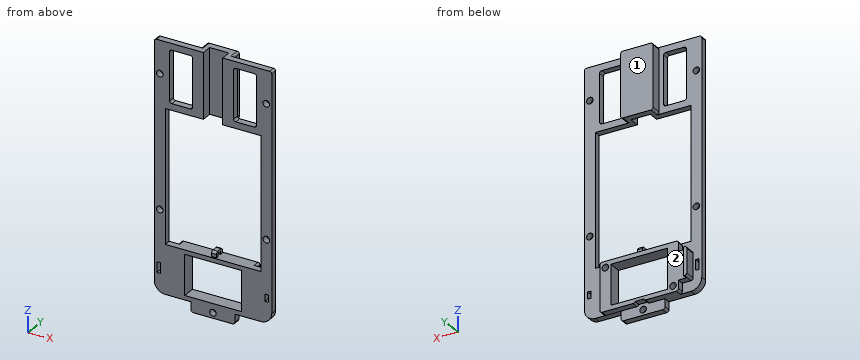
from build123d import *

# Parameters (mm, degrees)
BOSS_EXTRUDE1_DEPTH = 30
BOSS_EXTRUDE2_DEPTH = 3
SKETCH4_W           = 10.48
SKETCH4_H           = 24
CUT_EXTRUDE1_DEPTH  = 93.244717637
SKETCH5_R           = 1.5
CUT_EXTRUDE2_DEPTH  = 93.244717637
FILLET1_R           = 1
SKETCH7_W           = 26
SKETCH7_H           = 18.47
BOSS_EXTRUDE3_DEPTH = 3
SKETCH8_R           = 1.5
CUT_EXTRUDE3_DEPTH  = 4
SKETCH9_W           = 1.5
SKETCH9_H           = 13
BOSS_EXTRUDE4_DEPTH = 2
SKETCH10_W          = 26
SKETCH10_H          = 18.47
CUT_EXTRUDE4_DEPTH  = 3
SKETCH11_W          = 4
SKETCH11_H          = 0.67806633
CUT_EXTRUDE5_DEPTH  = 3
FILLET2_R           = 1
FILLET3_R           = 5
SKETCH12_W          = 1.6
SKETCH12_H          = 3.2
SKETCH12_H_2        = 4.8
CUT_EXTRUDE6_DEPTH  = 3
SKETCH13_W          = 2.25
SKETCH13_H          = 1.25
BOSS_EXTRUDE5_DEPTH = 1.5
SKETCH14_W          = 2.25
SKETCH14_H          = 4.5
BOSS_EXTRUDE6_DEPTH = 1
FILLET4_R           = 1


with BuildPart() as part:
    # Sketch1 → Boss-Extrude1 (new body)
    with BuildSketch(Plane.XY):
        Polygon((-26.9, 2.045135231), (-26.9, 5.045135231), (-7.42, 5.045135231), (-7.42, 9.845135231), (7.42, 9.845135231), (7.42, 5.045135231), (26.9, 5.045135231), (26.9, 2.045135231), (4.42, 2.045135231), (4.42, 6.845135231), (-4.42, 6.845135231), (-4.42, 2.045135231), align=None)
    extrude(amount=BOSS_EXTRUDE1_DEPTH)

    # Sketch3 → Boss-Extrude2 (add)
    with BuildSketch(Plane(origin=(0, 5.045135231, 0), x_dir=(1, 0, 0), z_dir=(0, 1, 0))):
        Polygon((26.9, 0), (26.9, 83.431524331), (10, 83.47), (10, 88.104698694), (-10.074836098, 88.104698694), (-10.074836098, 83.47), (-26.9, 83.47), (-26.9, 0), (-21.9, 0), (-21.9, 61), (21.9, 61), (21.9, 0), align=None)
    extrude(amount=-BOSS_EXTRUDE2_DEPTH)

    # Sketch4 → Cut-Extrude1 (cut, through all)
    with BuildSketch(Plane(origin=(0, 5.045135231, 0), x_dir=(1, 0, 0), z_dir=(0, 1, 0))):
        with Locations((14.66, -15)):
            Rectangle(SKETCH4_W, SKETCH4_H)
        with Locations((-14.66, -15)):
            Rectangle(SKETCH4_W, SKETCH4_H)
    extrude(amount=-CUT_EXTRUDE1_DEPTH, mode=Mode.SUBTRACT)

    # Sketch5 → Cut-Extrude2 (cut, through all)
    with BuildSketch(Plane(origin=(0, 5.045135231, 0), x_dir=(1, 0, 0), z_dir=(0, 1, 0))):
        with Locations(Location((24.4, -15, 0), (0, 0, 270))):
            Circle(SKETCH5_R)
        with Locations(Location((-24.4, -15, 0), (0, 0, 270))):
            Circle(SKETCH5_R)
        with Locations(Location((-0.037418049, 85.604698694, 0), (0, 0, 270))):
            Circle(SKETCH5_R)
        with Locations(Location((24.4, 46, 0), (0, 0, 270))):
            Circle(SKETCH5_R)
        with Locations(Location((-24.4, 46, 0), (0, 0, 270))):
            Circle(SKETCH5_R)
    extrude(amount=-CUT_EXTRUDE2_DEPTH, mode=Mode.SUBTRACT)

    # Fillet1
    fillet1_edges = [part.edges().sort_by_distance(p)[0] for p in [
        (-7.42, 7.445135231, 0),
        (7.42, 7.445135231, 0),
        (26.9, 3.545135231, 30),
        (7.42, 7.445135231, 30),
        (-10.074836098, 3.545135231, -88.104698694),
        (10, 3.545135231, -88.104698694),
        (-7.42, 7.445135231, 30),
        (-26.9, 3.545135231, 30),
        (9.42, 3.545135231, 27),
        (9.42, 3.545135231, 3),
        (19.9, 3.545135231, 3),
        (19.9, 3.545135231, 27),
        (-19.9, 3.545135231, 3),
        (-9.42, 3.545135231, 3),
        (-9.42, 3.545135231, 27),
        (-19.9, 3.545135231, 27),
    ]]
    fillet(fillet1_edges, radius=FILLET1_R)

    # Sketch7 → Boss-Extrude3 (add)
    with BuildSketch(Plane(origin=(0, 5.045135231, 0), x_dir=(1, 0, 0), z_dir=(0, 1, 0))):
        Polygon((-18, 83.47), (-18, 78.74462915), (-23, 78.74462915), (-23, 65.74462915), (-18, 65.74462915), (-18, 61), (18, 61), (18, 83.47), align=None)
        with Locations((0, 72.235)):
            Rectangle(SKETCH7_W, SKETCH7_H, mode=Mode.SUBTRACT)
    extrude(amount=BOSS_EXTRUDE3_DEPTH)

    # Sketch8 → Cut-Extrude3 (cut)
    with BuildSketch(Plane(origin=(0, 8.045135231, 0), x_dir=(1, 0, 0), z_dir=(0, 1, 0))):
        with Locations(Location((-15.5, 80.64462915, 0), (0, 0, 270))):
            Circle(SKETCH8_R)
        with Locations(Location((15.5, 63.84462915, 0), (0, 0, 270))):
            Circle(SKETCH8_R)
    extrude(amount=-CUT_EXTRUDE3_DEPTH, mode=Mode.SUBTRACT)

    # Sketch9 → Boss-Extrude4 (add)
    with BuildSketch(Plane(origin=(0, 8.045135231, 0), x_dir=(1, 0, 0), z_dir=(0, 1, 0))):
        with Locations((-22.25, 72.24462915)):
            Rectangle(SKETCH9_W, SKETCH9_H)
    extrude(amount=BOSS_EXTRUDE4_DEPTH)

    # Sketch10 → Cut-Extrude4 (cut)
    with BuildSketch(Plane(origin=(0, 5.045135231, 0), x_dir=(1, 0, 0), z_dir=(0, 1, 0))):
        with Locations((0, 72.235)):
            Rectangle(SKETCH10_W, SKETCH10_H)
    extrude(amount=-CUT_EXTRUDE4_DEPTH, mode=Mode.SUBTRACT)

    # Sketch11 → Cut-Extrude5 (cut)
    with BuildSketch(Plane(origin=(0, 8.045135231, 0), x_dir=(1, 0, 0), z_dir=(0, 1, 0))):
        with Locations((-0.037418049, 83.130966835)):
            Rectangle(SKETCH11_W, SKETCH11_H)
    extrude(amount=-CUT_EXTRUDE5_DEPTH, mode=Mode.SUBTRACT)

    # Fillet2
    # the kernel refuses this fillet: 1 mm, written as the material it takes off along each edge
    with BuildSketch(Plane(origin=(18, 5.045135231, -83.47), x_dir=(0, 0, 1), z_dir=(0, 1, 0)), Plane(origin=(-18, 5.045135231, -83.47), x_dir=(1, 0, 0), z_dir=(0, 1, 0)), Plane(origin=(-18, 5.045135231, -61), x_dir=(0, 0, -1), z_dir=(0, 1, 0)), Plane(origin=(18, 5.045135231, -61), x_dir=(-1, 0, 0), z_dir=(0, 1, 0))) as fillet2_piece_1:
        with BuildLine():
            CenterArc((FILLET2_R, -FILLET2_R), FILLET2_R, 90, 90)
            Line((0, -FILLET2_R), (-FILLET2_R * 0.02, -FILLET2_R))
            Line((-FILLET2_R * 0.02, -FILLET2_R), (-FILLET2_R * 0.02, FILLET2_R * 0.02))
            Line((-FILLET2_R * 0.02, FILLET2_R * 0.02), (FILLET2_R, FILLET2_R * 0.02))
            Line((FILLET2_R, FILLET2_R * 0.02), (FILLET2_R, 0))
        make_face()
    extrude(amount=5.5, mode=Mode.SUBTRACT)
    with BuildSketch(Plane(origin=(-23, 5.045135231, -78.74462915), x_dir=(1, 0, 0), z_dir=(0, 1, 0)), Plane(origin=(-23, 5.045135231, -65.74462915), x_dir=(0, 0, -1), z_dir=(0, 1, 0))) as fillet2_piece_2:
        with BuildLine():
            CenterArc((FILLET2_R, -FILLET2_R), FILLET2_R, 90, 90)
            Line((0, -FILLET2_R), (-FILLET2_R * 0.02, -FILLET2_R))
            Line((-FILLET2_R * 0.02, -FILLET2_R), (-FILLET2_R * 0.02, FILLET2_R * 0.02))
            Line((-FILLET2_R * 0.02, FILLET2_R * 0.02), (FILLET2_R, FILLET2_R * 0.02))
            Line((FILLET2_R, FILLET2_R * 0.02), (FILLET2_R, 0))
        make_face()
    extrude(amount=7.5, mode=Mode.SUBTRACT)
    with BuildSketch(Plane(origin=(1.962581951, 10.412040795, -83.47), x_dir=(1, 0, 0), z_dir=(0, -1, 0))) as fillet2_piece_3:
        with BuildLine():
            CenterArc((0.946762226, 1), FILLET2_R, 198.779905416, 71.220094584)
            Line((0, 0.67806633), (-0.018935245, 0.671627657))
            ThreePointArc((-0.018935245, 0.671627657), (-0.02, 0.339033165), (-0.02, 0))
            Line((-0.02, 0), (0, -0.02))
            Line((0, -0.02), (0.946762226, -0.02))
            Line((0.946762226, -0.02), (0.946762226, 0))
        make_face()
    extrude(amount=5.366905565, mode=Mode.SUBTRACT)
    with BuildSketch(Plane(origin=(-2.037418049, 10.412040795, -83.47), x_dir=(-1, 0, 0), z_dir=(0, -1, 0))) as fillet2_piece_4:
        with BuildLine():
            CenterArc((0.946762226, -1), FILLET2_R, 90, 71.220094584)
            Line((0, -0.67806633), (-0.018935245, -0.671627657))
            ThreePointArc((-0.018935245, -0.671627657), (-0.02, -0.339033165), (-0.02, 0))
            Line((-0.02, 0), (0, 0.02))
            Line((0, 0.02), (0.946762226, 0.02))
            Line((0.946762226, 0.02), (0.946762226, 0))
        make_face()
    extrude(amount=5.366905565, mode=Mode.SUBTRACT)

    # Fillet3
    fillet3_edges = [part.edges().sort_by_distance(p)[0] for p in [
        (-26.9, 3.545135231, -83.47),
        (26.9, 3.545135231, -83.431524331),
    ]]
    fillet(fillet3_edges, radius=FILLET3_R)

    # Sketch12 → Cut-Extrude6 (cut)
    with BuildSketch(Plane(origin=(0, 5.045135231, 0), x_dir=(1, 0, 0), z_dir=(0, 1, 0))):
        with Locations((24.6, 72.235)):
            Rectangle(SKETCH12_W, SKETCH12_H)
        with Locations((-24.85, 72.235)):
            Rectangle(SKETCH12_W, SKETCH12_H_2)
    extrude(amount=-CUT_EXTRUDE6_DEPTH, mode=Mode.SUBTRACT)

    # Sketch13 → Boss-Extrude5 (add)
    with BuildSketch(Plane.XY.offset(-61)):
        with Locations((0, 6.670135231)):
            Rectangle(SKETCH13_W, SKETCH13_H)
        with Locations((0, 3.420135231)):
            Rectangle(SKETCH13_W, SKETCH13_H)
    extrude(amount=BOSS_EXTRUDE5_DEPTH)

    # Sketch14 → Boss-Extrude6 (add)
    with BuildSketch(Plane.XY.offset(-59.5)):
        with Locations((0, 5.045135231)):
            Rectangle(SKETCH14_W, SKETCH14_H)
    extrude(amount=BOSS_EXTRUDE6_DEPTH)

    # Fillet4
    fillet4_edges = [part.edges().sort_by_distance(p)[0] for p in [
        (0, 2.795135231, -58.5),
        (0, 7.295135231, -58.5),
    ]]
    fillet(fillet4_edges, radius=FILLET4_R)


solid = part.part
Input: part model. Units: mm. Frame: model coordinates. Face numbers are marked on the shaded views. A direction names the side the tool comes from. Coordinates: 2 decimals unless noted, no trailing zeros. Order: outer loops, then holes, each group sorted by start corner. A loop starts at its lowest first (then second) coordinate and runs counter-clockwise, first axis right, second up. Notation, with made-up numbers: M -40,15 L 12,15 A9 cw 12,21 Z; hole C 31.5,35.5 d3. An arc over 180 degrees is marked long. Answer in a Markdown table with one row per item.
(1) Contact query for flat-ended pins moving along their axis: pin 1 Ø1 at (x, z) = (10.5, -61) entering from +Y; pin 2 Ø0.9 at (x, y) = (14.5, 3.5) entering from -Z; pin 3 Ø2 at (x, z) = (19.5, 13) entering from +Y. Output: stop coordinate, or through.
Numbers:
| item | result |
|---|---|
| pin 1 | stops at y = 8.05 |
| pin 2 | stops at z = -83.46 |
| pin 3 | stops at y = 5.05 |
(2) Section query D-D, the plane z = -46. Output: boundary loops of the cut face in (x, y).
Numbers:
| item | result |
|---|---|
| outline | M -26.9,2.05 L -25.9,2.05 L -25.9,5.05 L -26.9,5.05 Z; M -22.9,2.05 L -21.9,2.05 L -21.9,5.05 L -22.9,5.05 Z; M 21.9,2.05 L 22.9,2.05 L 22.9,5.05 L 21.9,5.05 Z; M 25.9,2.05 L 26.9,2.05 L 26.9,5.05 L 25.9,5.05 Z |
(3) Access query for the marked faces 1 and 2. Directions: +Z, -Z, +X, -X, +Y, -Y. A direction counts if a zero-diameter tool reaches every point of the face in a straight line with its end or side. Return the directions, or none.
Numbers:
| item | result |
|---|---|
| face 1 | +Z, -Z, +X, -X, +Y |
| face 2 | -Z, +X, +Y |
(4) Material intervals for line 1 (Z direction, x = 6.5, y = 6.25); line 2 (X direction, y = 3.45, z = -46); line 3 (X direction, y = 3.9, z = 15), sorted ascending. Write a range as [from, to].
Numbers:
| item | result |
|---|---|
| line 1 | z = [-83.47, -81.47], [-63, -61], [0, 30] |
| line 2 | x = [-26.9, -25.9], [-22.9, -21.9], [21.9, 22.9], [25.9, 26.9] |
| line 3 | x = [-26.9, -25.9], [-22.9, -19.9], [-9.42, -4.42], [4.42, 9.42], [19.9, 22.9], [25.9, 26.9] |
(5) Section query B-B, the plane x = -15.5. Output: boundary loops of the cut face in (y, z), plus the area to 3 significant figures.
Numbers:
| item | result |
|---|---|
| outline | M 2.05,-83.47 L 8.05,-83.47 L 8.05,-82.14 L 4.05,-82.14 L 4.05,-79.14 L 8.05,-79.14 L 8.05,-61 L 2.05,-61 Z; M 2.05,0 L 5.05,0 L 5.05,3 L 2.05,3 Z; M 2.05,27 L 5.05,27 L 5.05,30 L 2.05,30 Z |
| area | 141 mm^2 |
(6) Section query A-A, the plane z = 15. Output: boundary loops of the cut face in (x, y).
Numbers:
| item | result |
|---|---|
| outline | M -26.9,2.05 L -25.9,2.05 L -25.9,5.05 L -26.9,5.05 Z; M -22.9,2.05 L -19.9,2.05 L -19.9,5.05 L -22.9,5.05 Z; M -9.42,2.05 L -4.42,2.05 L -4.42,6.85 L 4.42,6.85 L 4.42,2.05 L 9.42,2.05 L 9.42,5.05 L 7.42,5.05 L 7.42,9.85 L -7.42,9.85 L -7.42,5.05 L -9.42,5.05 Z; M 19.9,2.05 L 22.9,2.05 L 22.9,5.05 L 19.9,5.05 Z; M 25.9,2.05 L 26.9,2.05 L 26.9,5.05 L 25.9,5.05 Z |
(7) Section query C-C, the plane z = -3.5. Output: boundary loops of the cut face in (x, y), plus the area to 3 significant figures.
Numbers:
| item | result |
|---|---|
| outline | M -26.9,2.05 L -21.9,2.05 L -21.9,5.05 L -26.9,5.05 Z; M 21.9,2.05 L 26.9,2.05 L 26.9,5.05 L 21.9,5.05 Z |
| area | 30.0 mm^2 |
